Design review of the part built by this model. Coordinates are the model's own, in mm. Face numbers are marked on the shaded views. A direction names the side the tool comes from. Coordinates: 2 decimals unless noted, no trailing zeros. Write each loop counter-clockwise with the first axis right and the second up, starting at its lowest first coordinate (ties: lowest second). Pieces come first, ordered by that corner, then holes. Notation, with made-up numbers: (66.5, 0) - (118.5, 0) arc R22 ccw to (118.5, 31) - close; hole circle Ø10 at (58.25, 49.25). An arc over 180 degrees is marked (long way). Answer as a JSON object with one key per item and string values.
```python
from build123d import *

# Parameters (mm, degrees)
SKETCH_R     = 35
PAD_DEPTH    = 30
SKETCH001_R  = 35
PAD001_DEPTH = 40
SKETCH002_R  = 37.5
POCKET_DEPTH = 35
PAD002_DEPTH = 10


with BuildPart() as part:
    # Sketch → Pad (new body)
    with BuildSketch(Plane.XY):
        Circle(SKETCH_R)
    extrude(amount=PAD_DEPTH)

    # Sketch001 → Pad001 (join)
    with BuildSketch(Plane.YZ):
        with Locations((0, 35)):
            Circle(SKETCH001_R)
    extrude(amount=-PAD001_DEPTH)

    # Sketch002 → Pocket (cut)
    with BuildSketch(Plane.YZ):
        with Locations((0, 35)):
            Circle(SKETCH002_R)
    extrude(amount=POCKET_DEPTH, mode=Mode.SUBTRACT)

    # Sketch → Pad002 (join)
    with BuildSketch(Plane.XY):
        Circle(SKETCH_R)
    extrude(amount=-PAD002_DEPTH)


solid = part.part
```
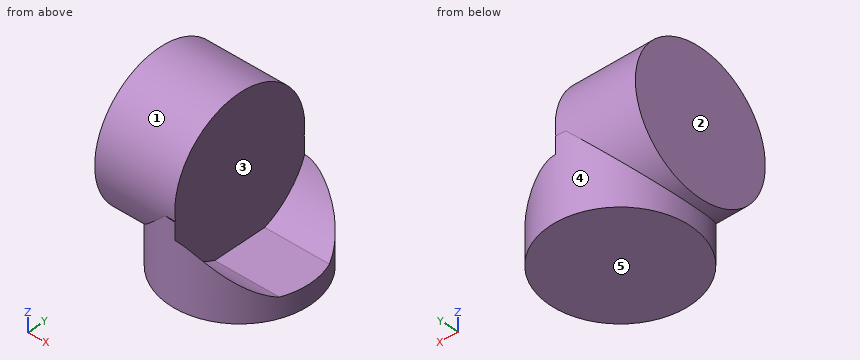
(1) Take a section at B-B, the plane z = 12. Write out the cut boundary in (x, y), and give its area (3 significant figures).
Solved:
{"outline": "(-40, -26.38) - (-23, -26.38) arc R35 ccw to (18.65, -29.62) - (0, -29.62) - (0, 29.62) - (18.65, 29.62) arc R35 ccw to (-23, 26.38) - (-40, 26.38) - close", "area": "2,520 mm^2"}
(2) Take a section at C-C, the plane x = 7. Write out the cut boundary in (y, z).
Solved:
{"outline": "(-34.29, -10) - (34.29, -10) - (34.29, 19.83) arc R37.5 cw to (13.46, 0) - (-13.46, 0) arc R37.5 cw to (-34.29, 19.83) - close"}
(3) To check wall thickness, follow line 1 (X direction, y = 9, z = 20); line 2 (Z direction, x = 20, y = 7); line 3 (Z direction, x = 3, y = -14.5). State the ranges of each line that lie inside material, in increasing order. Write a range as from..to.
Solved:
{"line 1": "x = -40..0", "line 2": "z = -10..0", "line 3": "z = -10..0.42"}
(4) Tool access review of the marked faces 1, 2, 3, 4 and 5: name each direction out of +Z, -Z, +X, -X, +Y, -Y from which nothing blocks a thin tool from reaching the whole face with its end or side.
Solved:
{"face 1": "-X", "face 2": "+Z, -Z, -X, +Y, -Y", "face 3": "+Z, +X", "face 4": "-Z", "face 5": "-Z, +X, -X, +Y, -Y"}
(5) Take a section at D-D, the plane z = 35. Write out the cut boundary in (x, y), and give its area (3 significant figures).
Solved:
{"outline": "(-40, -35) - (0, -35) - (0, 35) - (-40, 35) - close", "area": "2,800 mm^2"}
(6) For pin 1 (21 mm diameter, centred on y = -13.5, z = 44, fed in from +X); pin 2 (1 mm diameter, centred on x = -28, y = 5.5, fed in from +Z); pin 3 (8 mm diameter, centred on x = 18, y = 0.5, fed in from +Z), all flat-tipped, find the tip position at first contact; note any pin that passes through.
Solved:
{"pin 1": "stops at x = 0", "pin 2": "stops at z = 69.64", "pin 3": "stops at z = 0"}
(7) Take a section at A-A, the plane y = 0. Write out the cut boundary in (x, z), and give its area (3 significant figures).
Solved:
{"outline": "(-40, 0) - (-35, 0) - (-35, -10) - (35, -10) - (35, 0) - (0, 0) - (0, 70) - (-40, 70) - close", "area": "3,500 mm^2"}
